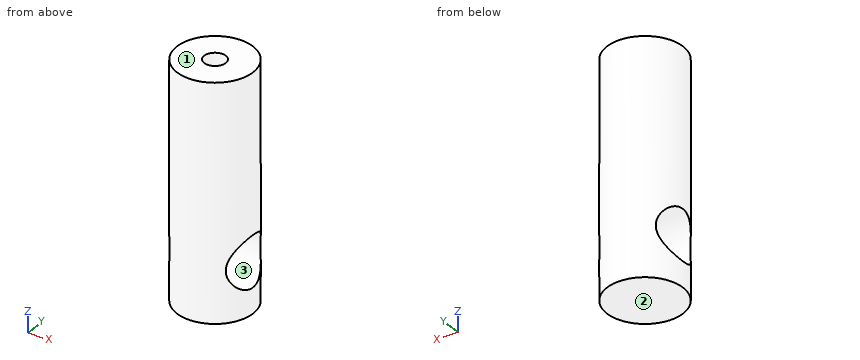
from build123d import *

# Parameters (mm, degrees)
SKETCH1_R                 = 4.7625
BOSS_EXTRUDE1_DEPTH       = 29.21
CUT_EXTRUDE2_DEPTH        = 30.97643929
CUT_EXTRUDE2_DEPTH_BACK   = 30.97643929
SKETCH3_R                 = 3.175
F_6_32_TAPPED_HOLE1_D     = 2.7051
F_6_32_TAPPED_HOLE1_DEPTH = 12.7
F_6_32_TAPPED_HOLE1_TIP   = 0.81269403


with BuildPart() as part:
    # Sketch1 → Boss-Extrude1 (new body)
    with BuildSketch(Plane.XY):
        Circle(SKETCH1_R)
    extrude(amount=BOSS_EXTRUDE1_DEPTH)

    # Sketch3 → Cut-Extrude2 (cut, two sides: drawn at the far end of the back side and taken through both)
    with BuildSketch(Plane(origin=(0, 0, 0), x_dir=(0, 0, -1), z_dir=(1, 0, 0)).offset(-CUT_EXTRUDE2_DEPTH_BACK)):
        with Locations((-6.35, 0)):
            Circle(SKETCH3_R)
    extrude(amount=CUT_EXTRUDE2_DEPTH + CUT_EXTRUDE2_DEPTH_BACK, mode=Mode.SUBTRACT)

    # #6-32 Tapped Hole1
    with Locations(Plane.XY.offset(29.21)):
        with Locations((0, 0)):
            Hole(F_6_32_TAPPED_HOLE1_D / 2, depth=F_6_32_TAPPED_HOLE1_DEPTH)
            with Locations((0, 0, -(F_6_32_TAPPED_HOLE1_DEPTH + F_6_32_TAPPED_HOLE1_TIP / 2))):  # 118° drill point
                Cone(0, F_6_32_TAPPED_HOLE1_D / 2, F_6_32_TAPPED_HOLE1_TIP, mode=Mode.SUBTRACT)


solid = part.part
Source: CAD feature listing. Evaluate the final solid. Frame: model axes, mm. Face numbers are marked on the shaded views. Coordinates: 2 decimals unless noted, no trailing zeros. Order: outer loops, then holes, each group sorted by start corner. A loop starts at its lowest first (then second) coordinate and runs counter-clockwise, first axis right, second up. Notation, with made-up numbers: M 32,27.5 L 46,27.5 A20 ccw 46,52.5 Z; hole C 12,21.25 d7. An arc over 180 degrees is marked long. Write each question's results on one line, items separated by ' | '. Start each with the question number.
1. Draft query along Z for the marked faces 1, 2 and 3. Return one class per face: +Z half, -Z half, draft (parallel to the pull), parting line (faces both ways), or undercut.
2. Section A-A, the plane x = 3.75. Return the cut outline in (y, z) (3 decimals).
3. Section D-D, the plane x = 2. Return the cut outline in (y, z) (3 decimals), then the cut area to 3 significant figures.
4. Pin query (flat end, axial travel): pin 1 (3 mm diameter, centred on x = 0.5, z = 20.5, fed in from +Y); pin 2 (1.5 mm diameter, centred on x = -2, z = 18.5, fed in from -Y); pin 3 (1.5 mm diameter, centred on y = -3.5, z = 25, fed in from +X). Return the tip coordinate at first contact, or that it passes through.
5. Material intervals for L1, parallel to X at y = 0, z = 20.5; L2, parallel to Z at x = -1.75, y = 1.25, sorted ascending.
6. Section C-C, the plane z = 21. Return the cut outline in (x, y) (1 decimal), then the cut area to 3 significant figures.
7. Section B-B, the plane y = 2.75. Return the cut outline in (x, z), then the cut area to 3 significant figures.
Solution:
1) face 1: +Z half | face 2: -Z half | face 3: undercut
2) outline: M -2.936,0 L 2.936,0 L 2.936,5.141 A3.175 cw -2.936,5.141 Z; M -2.936,7.559 A3.175 cw 2.936,7.559 L 2.936,29.21 L -2.936,29.21 Z
3) outline: M -4.322,0 L 4.322,0 L 4.322,29.21 L -4.322,29.21 Z; hole C 0,6.35 d6.35 | area: 221 mm²
4) pin 1: y = 4.76 | pin 2: y = -4.6 | pin 3: x = 3.89
5) L1: -4.76 to -1.35, 1.35 to 4.76 | L2: 0 to 3.43, 9.27 to 29.21
6) outline: C 0,0 d9.5; hole C 0,0 d2.7 | area: 65.5 mm²
7) outline: M -3.89,0 L 3.89,0 L 3.89,4.76 L -3.89,4.76 Z; M -3.89,7.94 L 3.89,7.94 L 3.89,29.21 L -3.89,29.21 Z | area: 202 mm²
